Geometry check sheet. Reference: the model listing, model coordinates, mm. A direction names the side the tool comes from. Coordinates: 2 decimals unless noted, no trailing zeros. Order: outer loops, then holes, each group sorted by start corner. A loop starts at its lowest first (then second) coordinate and runs counter-clockwise, first axis right, second up. Notation, with made-up numbers: M -1.75,77.25 L 27.25,77.25 A20 ccw 27.25,100.25 Z; hole C -1.5,7 d11. An arc over 180 degrees is marked long. One line per item, written item: value. Start each with the question number.
1) Go/stop test with flat-tipped pins: P1, Ø18, axis at x = 0, y = -30, coming from the -Z side; P2, Ø3, axis at y = -48.5, z = -10.5, coming from the +X side; P3, Ø1, axis at x = -11.5, y = -78, coming from the +Z side. Record where each tip stops, or that it passes through.
2) Sectioned sample at A-A, the plane y = -30. Enter the section's corners in (x, z).
3) Sectioned sample at C-C, the plane y = -64. Enter the section's corners in (x, z), then the cut area to 3 significant figures.
4) Access from +Z, -Z, +X, -X, +Y, -Y to the whole of each face (thin tool, end or side, straight path). Record for faces 4 (the cylindrical face through (22, -30, 26)), 5 (the cylindrical face through (8.306, -45.969, 27.535)), 6 (the cylindrical face through (-22, -30, 26)).
5) Sectioned sample at D-D, the plane y = 22. Enter the section's corners in (x, z), then the cut area to 3 significant figures.
6) Sectioned sample at B-B, the plane x = -13. State how many separate pieces and enclosed holes the cut face has, then the cut area to 3 significant figures.
7) Thickness scan on L1, parallel to Z at x = 0, y = 22; L2, parallel to Z at x = 24, y = -54.5; L3, parallel to Z at x = -12, y = -43.5. Record the ranges inside material, lowest first. Write a range as from..to.
8) Draft check along Z on faces 1 (the cylindrical face through (-3.905, -29.16, -29.745)), 2 (the flat face through (-4, -15, 25)), 3 (the cylindrical face through (23.846, -85.07, 7.509)). Enter one of: pulls with the +Z half, pulls with the -Z half, needs draft (parallel to the pull), parting line crosses it, or undercut.
Autodesk Inventor part; units mm, degrees
ref_plane "Plan de construction1" through (0, 0, 30) normal (0, 0, 1) x (1, 0, 0)
sketch "Esquisse2" plane through (0, 0, 0) normal (0, 0, 1) x (1, 0, 0)
  line L0 (0, 16.6667) -> (0, -18.8492)
  line L1 (0, 54) -> (0, -114) construction
  line L2 (30, 30) -> (25, 30)
  line L3 (25, 30) -> (25, 20)
  line L4 (25, 20) -> (23, 20)
  line L5 (23, 20) -> (15, 0)
  line L6 (15, 0) -> (15, -60)
  line L7 (15, -60) -> (23, -80)
  line L8 (23, -80) -> (25, -80)
  line L9 (25, -80) -> (25, -90)
  line L10 (25, -90) -> (30, -90)
  line L11 (30, -90) -> (30, 30)
  line L12 (-6, 0) -> (36, 0) construction
  dimension "d4" = 30
  dimension "d5" = 50
  dimension "d6" = 60
  dimension "d8" = 10
  dimension "d9" = 100
  dimension "d10" = 30
  dimension "d11" = 10
  dimension "d12" = 2
  dimension "d13" = 2
  dimension "d14" = 20
  dimension "d15" = 20
  dimension "d17" = 21.801
revolve "Révolution1" add sketch "Esquisse2" angle 360 about axis through (0, 16.6667, 0) along (0, -1, 0)
ref_plane "Plan de construction1" through (0, 0, 30) normal (0, 0, 1) x (1, 0, 0)
sketch "Esquisse3" plane through (0, 0, 30) normal (0, 0, 1) x (1, 0, 0)
  line L0 (-15, -60) -> (15, -60) construction
  line L1 (-15, 0) -> (-23, 20) construction
  line L2 (15, 0) -> (23, 20) construction
  line L3 (-32.34, 0) -> (32.34, 0) construction
  line L4 (-23, -80) -> (-15, -60) construction
  line L5 (23, -80) -> (15, -60) construction
  circle A0 centre (0, -30) radius 15
  line L6 (0, 40) -> (0, -100) construction
  line L7 (-15, -60) -> (-15, 0) construction
  line L8 (15, -60) -> (15, 0) construction
  point P0 (0, 0)
  dimension "d19" = 60
  dimension "d20" = 30
  dimension "d21" = 30
extrude "Extrusion1" cut sketch "Esquisse3" against normal blind 30
sketch "Esquisse4" plane through (0, 0, 30) normal (0, 0, 1) x (1, 0, 0)
  arc A0 (15, -30) -> (-15, -30) centre (0, -30) ccw construction
  arc A1 (-15, -30) -> (15, -30) centre (0, -30) ccw construction
  line L0 (-15, -60) -> (15, -60) construction
  line L1 (-15, 0) -> (15, 0) construction
  circle A2 centre (0, -30) radius 22
  circle A3 centre (0, -30) radius 15
  point P0 (0, 0)
  point P1 (0, -15)
  point P2 (0, -45)
  dimension "d24" = 44
extrude "Extrusion2" add sketch "Esquisse4" against normal blind 10
sketch "Esquisse6" plane through (0, 0, 30) normal (0, 0, 1) x (1, 0, 0)
  circle A0 centre (0, -30) radius 15 construction
  arc A1 (0, -8) -> (0, -52) centre (0, -30) ccw construction
  arc A2 (0, -52) -> (0, -8) centre (0, -30) ccw construction
  circle A3 centre (0, -30) radius 15
  circle A4 centre (0, -30) radius 18
  point P0 (0, 0)
  dimension "d27" = 36
extrude "Extrusion3" cut sketch "Esquisse6" against normal blind 5
properties part number "P007_CanonSupportRervoir"
Final values:
1. P1: stops at z = -30
1. P2: stops at x = 28.62
1. P3: stops at z = 27.91
2. outline: M -22,20.4 A30 ccw long 22,20.4 L 22,30 L 18,30 L 18,25 L 15,25 L 15,0 A15 cw -15,0 L -15,25 L -18,25 L -18,30 L -22,30 Z
3. outline: C 0,0 d60; hole C 0,0 d33.2
3. area: 1,960 mm^2
4. face 4: +Z, +X
4. face 5: +Z
4. face 6: +Z, -X
5. outline: C 0,0 d60; hole C 0,0 d50
5. area: 864 mm^2
6. separate pieces: 3
6. enclosed holes: 0
6. area: 3,360 mm^2
7. L1: z = -30..-25, 25..30
7. L2: z = -18..18
7. L3: z = -27.5..-9, 9..30
8. face 1: parting line crosses it
8. face 2: pulls with the +Z half
8. face 3: undercut
